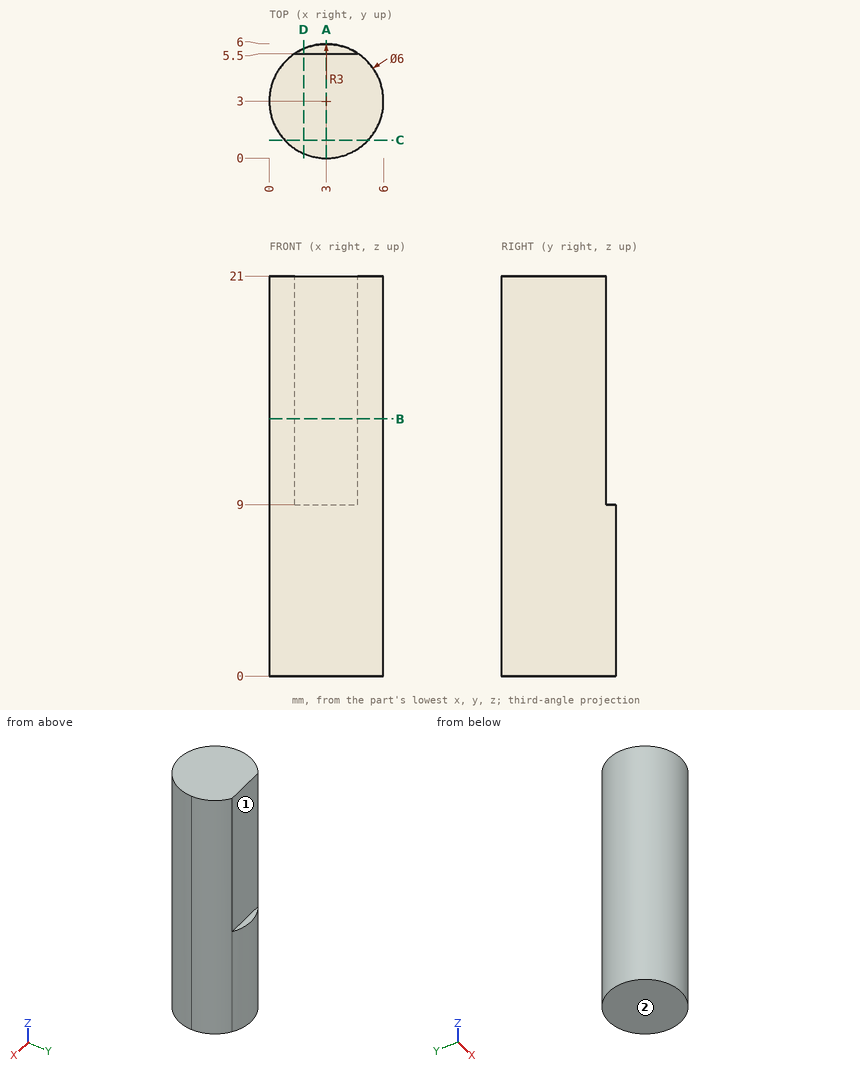
The drawing under review shows one solid part. Ordinate dimensions are in mm from its lowest x, y, z. A direction names the side the tool comes from. Round coordinates to 2 decimals unless told otherwise and drop trailing zeros. Loops run counter-clockwise (first coordinate to the right, second up) from the corner with the lowest first, then second, coordinate; pieces in that order, holes last. Notation, with made-up numbers: (-24, 50.25) - (-18, 50.25) arc R13 cw to (-18, 59.25) - close; hole circle Ø3 at (-25, 53.5). An arc over 180 degrees is marked (long way). Use a Markdown table: item, result. Add a question column.
Q1. Add section D-D (x = 1.8). State the section outline as (y, z) points, plus the area to 3 significant figures.
Q2. Add section C-C (y = 0.95). State the section outline as (x, z) points, plus the area to 3 significant figures.
Q3. Insertion check: pin 1 Ø2 at (x, y) = (1, 5) entering from -Z; pin 2 Ø1.5 at (y, z) = (0.5, 5) entering from +X; pin 3 Ø2.5 at (x, z) = (3, 15) entering from +Y. Each pin has a flat end and moves straight along its axis. Give the tip position at first contact, or say it passes through.
Q4. Add section A-A (x = 3). State the section outline as (y, z) points, plus the area to 3 significant figures.
Q5. Add section B-B (z = 13.5). State the section outline as (x, y) points.
Q6. Machinability: for the marked faces 1 and 2, which of the approach directions +Z, -Z, +X, -X, +Y, -Y give a long, thin tool a straight path to every point of the face, cutting with its end or side? Answer none if there is none.
Q7. For probe 1 along Y at (x, z) = (4.45, 4.75); probe 2 along Y at (x, z) = (1.95, 10); probe 3 along X at (y, z) = (1.7, 5.5), list the stretches that pass through material, from the lowest coordinate up.
Worked answers:
| question | item | result |
|---|---|---|
| 1 | outline | (0.25, 0) - (5.75, 0) - (5.75, 9) - (5.5, 9) - (5.5, 21) - (0.25, 21) - close |
| 1 | area | 112 mm² |
| 2 | outline | (0.81, 0) - (5.19, 0) - (5.19, 21) - (0.81, 21) - close |
| 2 | area | 92.0 mm² |
| 3 | pin 1 | z = 0 |
| 3 | pin 2 | x = 5.44 |
| 3 | pin 3 | y = 5.5 |
| 4 | outline | (0, 0) - (6, 0) - (6, 9) - (5.5, 9) - (5.5, 21) - (0, 21) - close |
| 4 | area | 120 mm² |
| 5 | outline | (1.34, 5.5) arc R3 ccw (long way) to (4.66, 5.5) - close |
| 6 | face 1 | +Z, +X, -X, +Y |
| 6 | face 2 | -Z, +X, -X, +Y, -Y |
| 7 | probe 1 | 0.37 to 5.63 |
| 7 | probe 2 | 0.19 to 5.5 |
| 7 | probe 3 | 0.3 to 5.7 |
